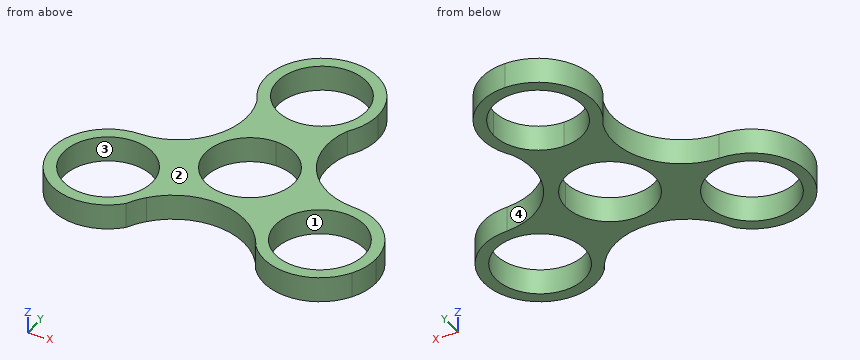
from build123d import *

# Parameters (mm, degrees)
F1_R     = 11.049
F2_DEPTH = 6.35
F4_DEPTH = 6.35
F0_R     = 44.45
F0_R_2   = 11.049
F5_DEPTH = 113
F7_DEPTH = 6.351


# Not quite as in the source:
# - an extrude ends at something that could not be found from the text; its depth is read off the source's solid


with BuildPart() as f2:
    # F1 (on face) → F2 (new body)
    with BuildSketch(Plane.XY):
        with BuildLine():
            ThreePointArc((11.2333605356, 22.1750309406), (6.2904881464, 18.0064015264), (0, 16.51))
            ThreePointArc((0, 16.51), (-6.2904881464, 18.0064015264), (-11.2333605356, 22.1750309406))
            ThreePointArc((-11.2333605356, 22.1750309406), (-12.7087939307, 6.5033813584), (-26.3964543073, -1.27))
            ThreePointArc((-26.3964543073, -1.27), (-16.5181725742, -5.3617182668), (-12.4264543073, -15.24))
            ThreePointArc((-12.4264543073, -15.24), (-12.7102714474, -18.0416599946), (-13.5501907032, -20.7294818894))
            ThreePointArc((-13.5501907032, -20.7294818894), (0.3483634498, -14.677920264), (13.8964774264, -21.477906538))
            ThreePointArc((13.8964774264, -21.477906538), (14.5157040294, -7.8909406838), (26.3964543073, -1.27))
            ThreePointArc((26.3964543073, -1.27), (12.7154911257, 6.507712775), (11.2333605356, 22.1750309406))
        make_face()
        with BuildLine():
            ThreePointArc((0, 13.97), (9.8782817332, 9.8782817332), (13.97, 0))
            ThreePointArc((13.97, 0), (-9.8782817332, -9.8782817332), (0, 13.97))
        make_face(mode=Mode.SUBTRACT)
        with BuildLine():
            ThreePointArc((-11.2333605356, 22.1750309406), (-6.2904881464, 18.0064015264), (0, 16.51))
            ThreePointArc((0, 16.51), (6.2904881464, 18.0064015264), (11.2333605356, 22.1750309406))
            ThreePointArc((11.2333605356, 22.1750309406), (13.2682128918, 26.1078807588), (13.97, 30.48))
            ThreePointArc((13.97, 30.48), (9.8782817686, 40.3582816978), (1.001e-07, 44.45))
            ThreePointArc((1.001e-07, 44.45), (-12.473598451, 36.7704881911), (-11.2333605356, 22.1750309406))
        make_face()
        with BuildLine():
            ThreePointArc((11.049, 30.48), (7.8128228253, 22.6671771747), (0, 19.431))
            ThreePointArc((0, 19.431), (-7.8128228253, 38.2928228253), (11.049, 30.48))
        make_face(mode=Mode.SUBTRACT)
        with BuildLine():
            ThreePointArc((-12.4264543073, -15.24), (-16.5181725742, -5.3617182668), (-26.3964543073, -1.27))
            ThreePointArc((-26.3964543073, -1.27), (-38.4948290673, -8.2549997732), (-38.4948294602, -22.2249995463))
            ThreePointArc((-38.4948294602, -22.2249995463), (-28.0548757974, -29.11121257), (-16.2857729321, -24.8802812266))
            ThreePointArc((-16.2857729321, -24.8802812266), (-15.0629921605, -22.709312564), (-13.5501907032, -20.7294818894))
            ThreePointArc((-13.5501907032, -20.7294818894), (-12.7102714474, -18.0416599946), (-12.4264543073, -15.24))
        make_face()
        with Locations((-26.3964543073, -15.24)):
            Circle(F1_R, mode=Mode.SUBTRACT)
        with BuildLine():
            ThreePointArc((40.3664543073, -15.24), (36.2747360405, -5.3617182668), (26.3964543073, -1.27))
            ThreePointArc((26.3964543073, -1.27), (14.5157040294, -7.8909406838), (13.8964774264, -21.477906538))
            ThreePointArc((13.8964774264, -21.477906538), (14.8325747733, -22.7814148116), (15.6479806578, -24.1636323436))
            ThreePointArc((15.6479806578, -24.1636323436), (27.5776113359, -29.1599773015), (38.4948290898, -22.2250001877))
            ThreePointArc((38.4948290898, -22.2250001877), (39.8904380726, -18.8557021648), (40.3664543073, -15.24))
        make_face()
        with Locations((26.3964543073, -15.24)):
            Circle(F1_R, mode=Mode.SUBTRACT)
    extrude(amount=F2_DEPTH)

    # F3 (on face) → F4 (join)
    with BuildSketch(Plane.XY):
        with BuildLine():
            ThreePointArc((0, 13.97), (-9.8782817332, -9.8782817332), (13.97, 0))
            ThreePointArc((13.97, 0), (9.8782817332, 9.8782817332), (0, 13.97))
        make_face()
        with BuildLine():
            ThreePointArc((11.049, 0), (-7.8128228253, -7.8128228253), (0, 11.049))
            ThreePointArc((0, 11.049), (7.8128228253, 7.8128228253), (11.049, 0))
        make_face(mode=Mode.SUBTRACT)
    extrude(amount=F4_DEPTH)

    # F0 (on Top) → F5 (cut, through all)
    with BuildSketch(Plane.XY):
        Circle(F0_R)
        with Locations((-26.3964543073, -15.24)):
            Circle(F0_R_2, mode=Mode.SUBTRACT)
        with Locations((26.3964543073, -15.24)):
            Circle(F0_R_2, mode=Mode.SUBTRACT)
        with BuildLine():
            ThreePointArc((0, 11.049), (7.8128228253, 7.8128228253), (11.049, 0))
            ThreePointArc((11.049, 0), (-7.8128228253, -7.8128228253), (0, 11.049))
        make_face(mode=Mode.SUBTRACT)
        with BuildLine():
            ThreePointArc((11.049, 30.48), (7.8128228253, 22.6671771747), (0, 19.431))
            ThreePointArc((0, 19.431), (-7.8128228253, 38.2928228253), (11.049, 30.48))
        make_face(mode=Mode.SUBTRACT)
    extrude(amount=-F5_DEPTH, mode=Mode.SUBTRACT)

    # F6 (on face) → F7 (cut, through all)
    with BuildSketch(Plane.XY.offset(6.35)):
        with BuildLine():
            Line((-26.3964543073, 15.7554745193), (-26.3964543073, -1.27))
            ThreePointArc((-26.3964543073, -1.27), (-12.7087939307, 6.5033813584), (-11.2333605356, 22.1750309406))
            Line((-11.2333605356, 22.1750309406), (-26.3964543073, 15.7554745193))
        make_face()
    extrude(amount=-F7_DEPTH, mode=Mode.SUBTRACT)


solid = f2.part
Design review of the part built by this model. Coordinates are the model's own, in mm. Face numbers are marked on the shaded views. Coordinates: 2 decimals unless noted, no trailing zeros. Write each loop counter-clockwise with the first axis right and the second up, starting at its lowest first coordinate (ties: lowest second). Pieces come first, ordered by that corner, then holes. Notation, with made-up numbers: (-28, 33) -> (31, 33) arc R22 ccw to (31, 57) -> close; hole circle Ø3 at (18.5, 21.5). An arc over 180 degrees is marked (long way). Write each question's results on one line, items separated by ' | '. Start each with the question number.
(1) Take a section at A-A on x = 25. Write out the cut boundary in (y, z).
(2) Take a section at B-B on z = 4.5. Write out the cut boundary in (x, y) (3 decimals), and give its area (3 significant figures).
(3) The part is to be moulded in two halves that separate along X. For the marked faces 1, 2, 3 and 4, say which applies: pulls with the +X half, pulls with the -X half, needs draft (parallel to the pull), parting line crosses it, or undercut.
(4) Take a section at C-C on x = 5. Write out the cut boundary in (y, z), and give its area (3 significant figures).
(5) For line 1 along Y through (x, z) = (-0.5, 1.5); line 2 along X through (y, z) = (-10, 2); line 3 along Y through (x, z) = (-5.5, 0.75), list the stretches that pass through material, from the lowest coordinate up. Write a range as from..to.
(6) Take a section at D-D on x = -28.5. Write out the cut boundary in (y, z), and give its area (3 significant figures).
(7) Clearance check with flat-ended pins moving along their axes: P1, Ø1, axis at x = -32, z = 2, coming from the +Y side; P2, Ø1, axis at y = 4, z = 1, coming from the +X side; P3, Ø1.5, axis at x = -7, z = 1, coming from the -Y side. State where each tip first meets the part, or that it passes through.
Results found:
1) outline: (-29.14, 0) -> (-26.2, 0) -> (-26.2, 6.35) -> (-29.14, 6.35) -> close; (-4.28, 0) -> (-1.16, 0) -> (-1.16, 6.35) -> (-4.28, 6.35) -> close
2) outline: (-26.396, -1.27) arc R13.97 ccw (long way) to (-16.286, -24.88) arc R17.874 cw to (15.648, -24.164) arc R13.97 ccw (long way) to (26.396, -1.27) arc R17.047 cw to (11.233, 22.175) arc R13.97 ccw (long way) to (-11.233, 22.175) arc R17.037 cw to start; hole circle Ø22.098 at (-26.396, -15.24); hole circle Ø22.098 at (0, 0); hole circle Ø22.098 at (0, 30.48); hole circle Ø22.098 at (26.396, -15.24) | area: 1,270 mm2
3) face 1: undercut | face 2: needs draft | face 3: undercut | face 4: pulls with the +X half
4) outline: (-15.43, 0) -> (-9.85, 0) -> (-9.85, 6.35) -> (-15.43, 6.35) -> close; (9.85, 0) -> (20.63, 0) -> (20.63, 6.35) -> (9.85, 6.35) -> close; (40.33, 0) -> (43.52, 0) -> (43.52, 6.35) -> (40.33, 6.35) -> close | area: 124 mm2
5) line 1: y = -14.67..-11.04, 11.04..19.44, 41.52..44.44 | line 2: x = -39.35..-36.12, -16.67..-4.7, 4.7..16.67, 36.12..39.35 | line 3: y = -15.49..-9.58, 9.58..20.9, 40.06..43.32
6) outline: (-29.05, 0) -> (-26.09, 0) -> (-26.09, 6.35) -> (-29.05, 6.35) -> close; (-4.39, 0) -> (-1.43, 0) -> (-1.43, 6.35) -> (-4.39, 6.35) -> close | area: 37.6 mm2
7) P1: stops at y = -2.24 | P2: stops at x = 15.19 | P3: stops at y = -16.37
